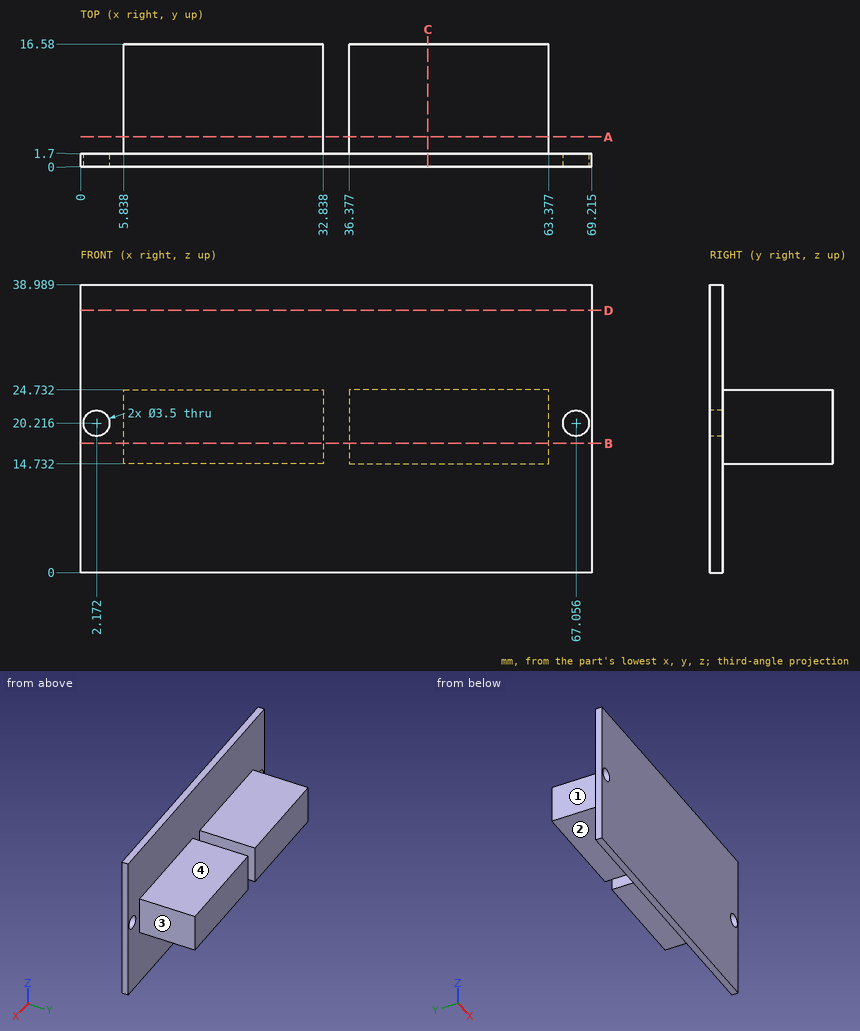
The drawing under review shows one solid part. Ordinate dimensions are in mm from its lowest x, y, z. A direction names the side the tool comes from. Give positions to 0.01 mm unless a question says otherwise; leave off trailing zeros. Order: outer loops, then holes, each group sorted by start corner. A loop starts at its lowest first (then second) coordinate and runs counter-clockwise, first axis right, second up. Notation, with made-up numbers: M 71.5,69.25 L 110.5,69.25 A33 cw 110.5,108.25 Z; hole C 28,8.5 d1. An arc over 180 degrees is marked long. One line per question, with ' | ' between items. Start each with the question number.
Q1. For pin 1 Ø3 at (y, z) = (7.5, 17.5) entering from +X; pin 2 Ø3 at (x, z) = (14, 12.5) entering from +Y; pin 3 Ø3 at (x, z) = (67.056, 20.216) entering from +Y; pin 4 Ø4.5 at (x, y) = (54, 9.5) entering from +Z, all flat-tipped, find the tip position at first contact; note any pin that passes through.
Q2. We need section C-C (x = 47). Write out the cut boundary in (y, z), plus the area to 3 significant figures.
Q3. For L1, parallel to X at y = 5, z = 21; L2, parallel to X at y = 1, z = 19.5 (3 decimals); L3, parallel to Y at x = 14.5, z = 32, list the stretches that pass through material, from the lowest coordinate up. Write a range as [from, to].
Q4. We need section B-B (z = 17.5). Write out the cut boundary in (x, y) (3 decimals).
Q5. We need section A-A (y = 4). Write out the cut boundary in (x, z), plus the area to 3 significant figures.
Q6. Machinability: for the marked faces 1, 2, 3 and 4, which of the approach directions +Z, -Z, +X, -X, +Y, -Y give a long, thin tool a straight path to every point of the face, cutting with its end or side? Answer none if there is none.
Q7. We need section D-D (z = 35.5). Write out the cut boundary in (x, y) (3 decimals), plus the area to 3 significant figures.
Returned:
1) pin 1: x = 63.38 | pin 2: y = 1.7 | pin 3: through | pin 4: z = 24.73
2) outline: M 0,0 L 1.7,0 L 1.7,14.73 L 16.58,14.73 L 16.58,24.73 L 1.7,24.73 L 1.7,38.99 L 0,38.99 Z | area: 215 mm2
3) L1: [5.84, 32.84], [36.38, 63.38] | L2: [0, 0.575], [3.769, 65.459], [68.653, 69.215] | L3: [0, 1.7]
4) outline: M 0,0 L 69.215,0 L 69.215,1.7 L 63.377,1.7 L 63.377,16.58 L 36.377,16.58 L 36.377,1.7 L 32.838,1.7 L 32.838,16.58 L 5.838,16.58 L 5.838,1.7 L 0,1.7 Z
5) outline: M 5.84,14.73 L 32.84,14.73 L 32.84,24.73 L 5.84,24.73 Z; M 36.38,14.73 L 63.38,14.73 L 63.38,24.73 L 36.38,24.73 Z | area: 540 mm2
6) face 1: +Z, -Z, -X, +Y | face 2: -Z, +X, -X, +Y | face 3: +Z, -Z, +X, +Y | face 4: +Z, +X, -X, +Y
7) outline: M 0,0 L 69.215,0 L 69.215,1.7 L 0,1.7 Z | area: 118 mm2
